Geometry check sheet. Reference: the model listing, model coordinates, mm. A direction names the side the tool comes from. Round coordinates to 2 decimals unless told otherwise and drop trailing zeros. Write each loop counter-clockwise with the first axis right and the second up, starting at its lowest first coordinate (ties: lowest second). Pieces come first, ordered by that corner, then holes. Notation, with made-up numbers: M -22,-15 L -4,-15 A17 cw -4,2 Z; hole C 27,55 d11. An arc over 180 degrees is marked long. Answer as CSV lines item,"result". Start each with the question number.
```python
from build123d import *

# Parameters (mm, degrees)
BOSS_EXTRUDE1_DEPTH = 15
SKETCH3_W           = 3
SKETCH3_H           = 0.5
CUT_EXTRUDE1_DEPTH  = 1
SKETCH2_W           = 3
SKETCH2_H           = 0.5
CUT_EXTRUDE2_DEPTH  = 1
SKETCH5_R           = 0.5
CUT_EXTRUDE3_DEPTH  = 0.25


with BuildPart() as part:
    # Sketch1 → Boss-Extrude1 (new body, symmetric)
    with BuildSketch(Plane.XY):
        Polygon((0, 0), (17, 0), (17, 1), (1, 1), (1, 31), (17, 31), (17, 32), (0, 32), align=None)
    extrude(amount=BOSS_EXTRUDE1_DEPTH, both=True)

    # Sketch3 → Cut-Extrude1 (cut)
    with BuildSketch(Plane(origin=(17, 0, 0), x_dir=(0, 0, -1), z_dir=(1, 0, 0))):
        with Locations((0, 0.495)):
            Rectangle(SKETCH3_W, SKETCH3_H)
    extrude(amount=-CUT_EXTRUDE1_DEPTH, mode=Mode.SUBTRACT)

    # Sketch2 → Cut-Extrude2 (cut)
    with BuildSketch(Plane(origin=(17, 0, 0), x_dir=(0, 0, -1), z_dir=(1, 0, 0))):
        with Locations((0, 31.5)):
            Rectangle(SKETCH2_W, SKETCH2_H)
    extrude(amount=-CUT_EXTRUDE2_DEPTH, mode=Mode.SUBTRACT)

    # Sketch5 → Cut-Extrude3 (cut, symmetric)
    with BuildSketch(Plane.ZY):
        with Locations((0, 16)):
            Circle(SKETCH5_R)
    extrude(amount=CUT_EXTRUDE3_DEPTH, both=True, mode=Mode.SUBTRACT)


solid = part.part
```
1) Section check C-C, the plane z = 0. Record the cut outline in (x, y) (3 decimals).
2) Mould release check, pull along Z, two halves, no side actions. Record for faces 4 (the flat face through (0, 16, 4)), 5 (the flat face through (16.5, 0.745, 0)), 6 (the flat face through (16.5, 31.75, 0)), 7 (the flat face through (0.3, 16.1, 15)): released by +Z, released by -Z, zero draft, split by the parting line, or undercut.
3) Scan lines: line 1 (Y direction, x = 4.5, z = -9.5); line 2 (Y direction, x = 0.1, z = 0); line 3 (X direction, y = 16, z = -12.5). Record each from-to range of solid material in increasing order. Write a range as from..to.
4) Go/stop test with flat-tipped pins: pin 1 (12 mm diameter, centred on y = 17, z = 1.5, fed in from +X); pin 2 (2 mm diameter, centred on x = 3, y = 19.5, fed in from -Z). Record where each tip stops, or that it passes through.
5) Section check D-D, the plane y = 21. Record the cut outline in (x, z).
6) Section check A-A, the plane x = 3. Record the cut outline in (y, z), plus the area to 3 significant figures.
7) Access from +Z, -Z, +X, -X, +Y, -Y to the whole of each face (thin tool, end or side, straight path). Record for faces 1 (the flat face through (16.5, 31.25, 0)), 2 (the flat face through (9, 1, 0)), 3 (the flat face through (0.25, 16, 0)).
8) Section check B-B, the plane y = 16. Record the cut outline in (x, z), plus the area to 4 significant figures.
Results:
1,outline,"M 0,0 L 17,0 L 17,0.245 L 16,0.245 L 16,0.745 L 17,0.745 L 17,1 L 1,1 L 1,31 L 17,31 L 17,31.25 L 16,31.25 L 16,31.75 L 17,31.75 L 17,32 L 0,32 L 0,16.5 L 0.25,16.5 L 0.25,15.5 L 0,15.5 Z"
2,face 4,"zero draft"
2,face 5,"undercut"
2,face 6,"undercut"
2,face 7,"released by +Z"
3,line 1,"y = 0..1, 31..32"
3,line 2,"y = 0..15.5, 16.5..32"
3,line 3,"x = 0..1"
4,pin 1,"stops at x = 1"
4,pin 2,"passes through"
5,outline,"M 0,-15 L 1,-15 L 1,15 L 0,15 Z"
6,outline,"M 0,-15 L 1,-15 L 1,15 L 0,15 Z; M 31,-15 L 32,-15 L 32,15 L 31,15 Z"
6,area,"60.0 mm^2"
7,face 1,"+X"
7,face 2,"+Z, -Z, +X"
7,face 3,"-X"
8,outline,"M 0,-15 L 1,-15 L 1,15 L 0,15 L 0,0.5 L 0.25,0.5 L 0.25,-0.5 L 0,-0.5 Z"
8,area,"29.75 mm^2"
